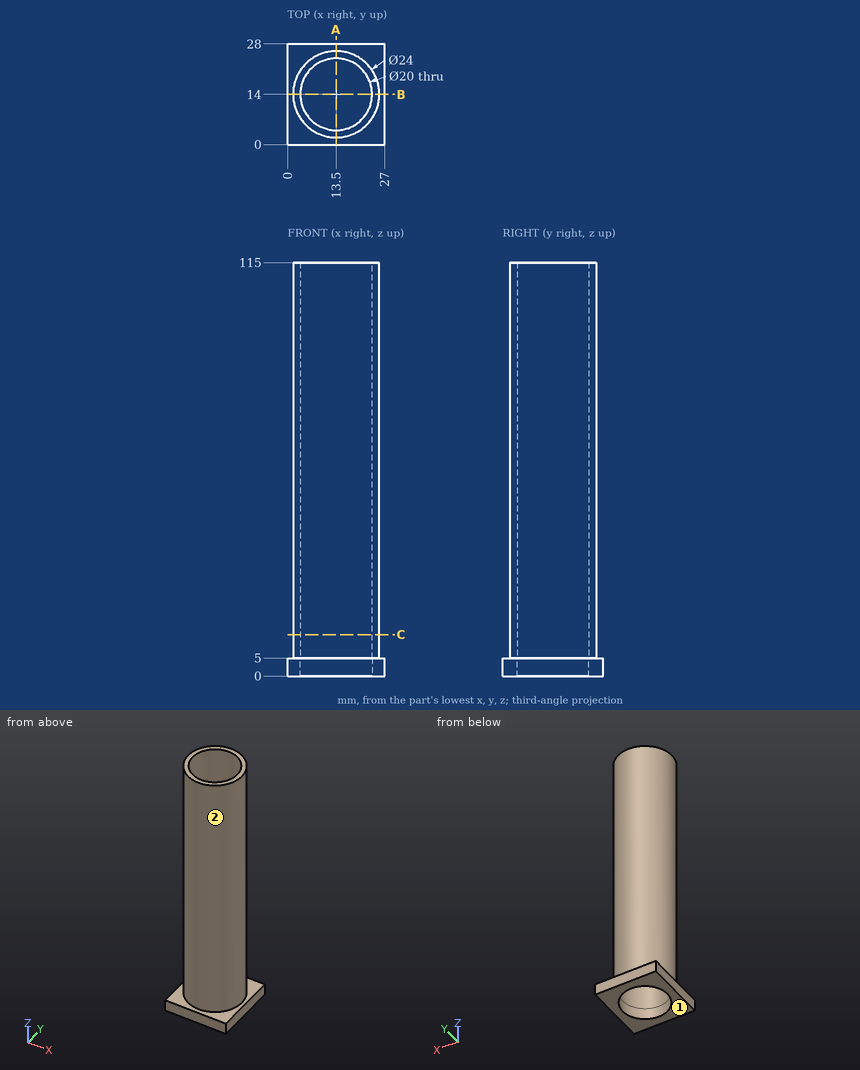
Can you work these out from the drawing? Everything is in mm from the part's minimum corner. A direction names the side the tool comes from. Round coordinates to 2 decimals unless told otherwise and drop trailing zeros. Write each loop counter-clockwise with the first axis right and the second up, starting at its lowest first coordinate (ties: lowest second). Pieces come first, ordered by that corner, then holes. Notation, with made-up numbers: (31.5, -32) - (47.5, -32) arc R27 cw to (47.5, 1) - close; hole circle Ø6 at (8, -17). An arc over 180 degrees is marked (long way). Use a Markdown table: item, result.
Q1. For the marked faces 1 and 2, which set-ups out of +Z, -Z, +X, -X, +Y, -Y let a thin tool reach every point of the face, with its end or its side?
Output values:
| item | result |
|---|---|
| face 1 | -Z, +X, -X, +Y, -Y |
| face 2 | +Z |
Q2. I want a section at C-C (z = 11.5). List the corners of the cut face in (x, y) for me.
Output values:
| item | result |
|---|---|
| outline | circle Ø24 at (13.5, 14); hole circle Ø20 at (13.5, 14) |
Q3. For pin 1 (6 mm diameter, centred on x = 24, z = 102.5, fed in from +Y); pin 2 (3 mm diameter, centred on x = 22.5, z = 68, fed in from -Y); pin 3 (3 mm diameter, centred on x = 17.5, z = 30, fed in from -Y); pin 4 (16 mm diameter, centred on x = 13.5, y = 14, fed in from +Z), each with a flat end and sliding along its axis, tell me the tip position at first contact or that it passes through.
Output values:
| item | result |
|---|---|
| pin 1 | y = 23.37 |
| pin 2 | y = 4.63 |
| pin 3 | y = 2.26 |
| pin 4 | through |
Q4. I want a section at A-A (x = 13.5). List the corners of the cut face in (y, z) for me, plus the area to 3 significant figures.
Output values:
| item | result |
|---|---|
| outline | (0, 0) - (4, 0) - (4, 115) - (2, 115) - (2, 5) - (0, 5) - close; (24, 0) - (28, 0) - (28, 5) - (26, 5) - (26, 115) - (24, 115) - close |
| area | 480 mm2 |
Q5. I want a section at B-B (y = 14). List the corners of the cut face in (x, z) for me.
Output values:
| item | result |
|---|---|
| outline | (0, 0) - (3.5, 0) - (3.5, 115) - (1.5, 115) - (1.5, 5) - (0, 5) - close; (23.5, 0) - (27, 0) - (27, 5) - (25.5, 5) - (25.5, 115) - (23.5, 115) - close |
Q6. Please list where these lines run through material, in increasing order: L1, parallel to Y at x = 13.5, z = 1.8; L2, parallel to Y at x = 13.5, z = 60.5; L3, parallel to Z at x = 3.5, y = 6.
Output values:
| item | result |
|---|---|
| L1 | 0 to 4, 24 to 28 |
| L2 | 2 to 4, 24 to 26 |
| L3 | 0 to 5 |
